Autodesk Inventor part; units mm, degrees
ref_plane "YZ Plane" through (0, 0, 0) normal (1, 0, 0) x (0, 1, 0)
ref_plane "XZ Plane" through (0, 0, 0) normal (0, 1, 0) x (-1, 0, 0)
ref_plane "XY Plane" through (0, 0, 0) normal (0, 0, 1) x (1, 0, 0)
sketch "Sketch1" plane through (0, 0, 0) normal (0, 0, 1) x (1, 0, 0)
  line L0 (-44, -62.5) -> (44, -62.5)
  line L1 (44, -62.5) -> (44, 62.5)
  line L2 (44, 62.5) -> (-44, 62.5)
  line L3 (-44, 62.5) -> (-44, -62.5)
  line L4 (-44, -62.5) -> (44, 62.5) construction
  line L5 (44, -62.5) -> (-44, 62.5) construction
  line L6 (35, 57.5) -> (-33, 57.5)
  line L7 (-33, 57.5) -> (-33, -34.5)
  line L8 (-33, -34.5) -> (35, -34.5)
  line L9 (35, -34.5) -> (35, 57.5)
  point P0 (0, 0)
  dimension "d154" = 88
  dimension "d155" = 125
  dimension "d185" = 68
  dimension "d186" = 92
  dimension "d187" = 11
  dimension "d188" = 9
  dimension "d190" = 5
extrude "Plate5" add sketch "Sketch1" along normal blind 2
sketch "Sketch7" plane through (-42, -62.5, 0) normal (-1, 0, 0) x (0, -1, 0)
  line L0 (-125, 0) -> (0, 0)
  line L1 (0, 0) -> (0, 90)
  line L2 (0, 90) -> (-125, 90)
  line L3 (-125, 90) -> (-125, 0)
edge flange "Flange3" height 90 angle 90 thickness 2 bend radius 2.75 thickness toward (-1, 0, 0) relief round relief width 2 relief depth 1 edges at (-44, 0, 2) wall of the first edge with corners at (-42, 62.5, 0) (-42, -62.5, 0) (-42, -62.5, 90) (-42, 62.5, 90)
bend "Bend3"
corner "Corner3"
sketch "Sketch9" plane through (-44, -62.5, 90) normal (-1, 0, 0) x (0, 0, 1)
  line L0 (-27.375, 69.75) -> (-57.875, 69.75)
  line L1 (-57.875, 69.75) -> (-57.875, 100.25)
  line L2 (-57.875, 100.25) -> (-27.375, 100.25)
  line L3 (-27.375, 100.25) -> (-27.375, 69.75)
  line L4 (-27.375, 69.75) -> (-57.875, 100.25) construction
  line L5 (-57.875, 69.75) -> (-27.375, 100.25) construction
  circle A0 centre (-19.625, 62) radius 2.5
  circle A1 centre (-65.625, 62) radius 2.5
  circle A2 centre (-65.625, 108) radius 2.5
  circle A3 centre (-19.625, 108) radius 2.5
  circle A4 centre (-42.625, 85) radius 32.5269 construction
  line L6 (-57.875, 69.75) -> (-65.625, 62) construction
  line L7 (-17.125, 59.5) -> (-68.125, 59.5) construction
  line L8 (-68.125, 59.5) -> (-68.125, 110.5) construction
  line L9 (-68.125, 110.5) -> (-17.125, 110.5) construction
  line L10 (-17.125, 110.5) -> (-17.125, 59.5) construction
  line L11 (-17.125, 59.5) -> (-68.125, 110.5) construction
  line L12 (-68.125, 59.5) -> (-17.125, 110.5) construction
  line L13 (-85.25, 125) -> (0, 125)
  line L14 (-42.625, 125) -> (-42.625, 85) construction
  circle A5 centre (-65.625, 108) radius 10.9602 construction
  line L15 (-19.625, 62) -> (-65.625, 62) construction
  line L16 (-65.625, 62) -> (-65.625, 108) construction
  line L17 (-65.625, 108) -> (-19.625, 108) construction
  line L18 (-19.625, 108) -> (-19.625, 62) construction
  line L19 (-19.625, 62) -> (-65.625, 108) construction
  line L20 (-65.625, 62) -> (-19.625, 108) construction
  point P0 (-90, 62.5)
  point P1 (-104.8197, 150.8767)
  point P2 (-104.8197, 150.8767)
  dimension "d181" = 21.9203
  dimension "d174" = 30.5
  dimension "d175" = 30.5
  dimension "d176" = 5
  dimension "d179" = 40
  dimension "d180" = 51
  dimension "d184" = 46
cut "Cut2" [suppressed]
properties part number "PRS 1652 DrSysB Central tube wall_D1200" material "Stainless Steel"
Can you work these out from the model? Positions are in its coordinate system, mm. A direction names the side the tool comes from. Give positions to 0.01 mm unless a question says otherwise; leave off trailing zeros. Order: outer loops, then holes, each group sorted by start corner. A loop starts at its lowest first (then second) coordinate and runs counter-clockwise, first axis right, second up. Notation, with made-up numbers: M -34.75,78.25 L 13.25,78.25 A19 ccw 13.25,110.25 Z; hole C -11.5,78.5 d6. An arc over 180 degrees is marked long. Use a Markdown table: item, result. Add a question column.
Item 1: Suppose I cut it at D-D (z = 22). List the corners of the cut face in (x, y) for me.
Item 2: If I drill on L1, parallel to X at y = -20, z = 59.5; L2, parallel to Z at x = -35.5, y = -54.5, over which ranges is the centre line in solid material (lowest first)? Write a range as [from, to].
Item 3: Suppose I cut it at C-C (y = -37). List the corners of the cut face in (x, z) for me, then the cut area to 3 significant figures.
Item 4: Suppose I cut it at A-A (x = 2.5). List the corners of the cut face in (y, z) for me, then the cut area to 3 significant figures.
Item 5: Will these pins go through, and if not, where does the flat tip stop? pin 1 (8 mm diameter, centred on y = 30, z = 44.5, fed in from +X); pin 2 (1.6 mm diameter, centred on y = 29.5, z = 1.5, fed in from -X).
Item 6: Suppose I cut it at B-B (y = 51.5). List the corners of the cut face in (x, z) for me.
Item 7: For faces 1 (the flat face through (2, -41, 0)), 2 (the flat face through (2, -41, 2)), which set-ups out of +Z, -Z, +X, -X, +Y, -Y let a thin tool reach every point of the face, with its end or its side?
Answer sheet:
| question | item | result |
|---|---|---|
| 1 | outline | M -44,-62.5 L -42,-62.5 L -42,62.5 L -44,62.5 Z |
| 2 | L1 | x = [-44, -42] |
| 2 | L2 | z = [0, 2] |
| 3 | outline | M -44,4.75 A4.75 ccw -39.25,0 L 44,0 L 44,2 L -39.25,2 A2.75 cw -42,4.75 L -42,90 L -44,90 Z |
| 3 | area | 349 mm² |
| 4 | outline | M -62.5,0 L -34.5,0 L -34.5,2 L -62.5,2 Z; M 57.5,0 L 62.5,0 L 62.5,2 L 57.5,2 Z |
| 4 | area | 66.0 mm² |
| 5 | pin 1 | stops at x = -42 |
| 5 | pin 2 | stops at x = -43.32 |
| 6 | outline | M -44,4.75 A4.75 ccw -39.25,0 L -33,0 L -33,2 L -39.25,2 A2.75 cw -42,4.75 L -42,90 L -44,90 Z; M 35,0 L 44,0 L 44,2 L 35,2 Z |
| 7 | face 1 | -Z, +X, -X, +Y, -Y |
| 7 | face 2 | +Z, +X, +Y, -Y |
